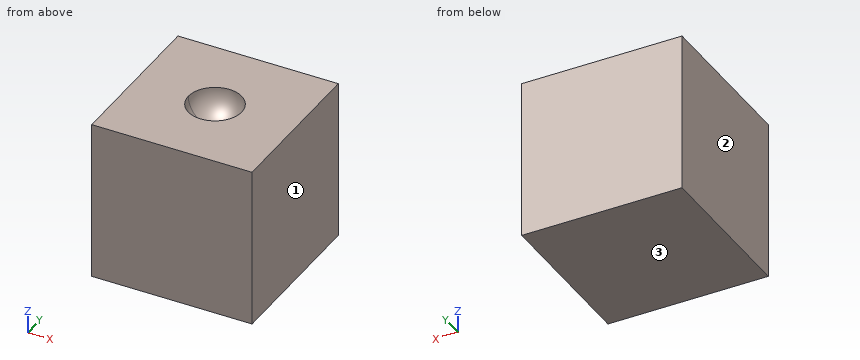
from build123d import *
from build123d.topology import SkipClean

# Parameters (mm, degrees)
SKETCH1_W           = 18
SKETCH1_H           = 18
BOSS_EXTRUDE1_DEPTH = 18


with BuildPart() as part:
    # Sketch1 → Boss-Extrude1 (new body)
    with BuildSketch(Plane.XY):
        Rectangle(SKETCH1_W, SKETCH1_H)
    extrude(amount=BOSS_EXTRUDE1_DEPTH)

    # Sketch2 → Cut-Revolve1 (revolve, cut)
    with SkipClean():  # the faces are left unmerged after this step: merging them gives an invalid solid
        with BuildSketch(Plane.XY.offset(18)):
            with BuildLine():
                ThreePointArc((3, 0), (2.121320344, 2.121320344), (0, 3))
                Line((0, 3), (0, -3))
                ThreePointArc((0, -3), (2.121320344, -2.121320344), (3, 0))
            make_face()
            with BuildLine():
                Line((0, -3), (0, 3))
                ThreePointArc((0, 3), (-3, 0), (0, -3))
            make_face()
        revolve(axis=Axis((0, 3, 18), (0, -1, 0)), mode=Mode.SUBTRACT)


solid = part.part
CAD build for the part. Positions are in the model's coordinates, mm. Face numbers are marked on the shaded views. Round coordinates to 2 decimals unless told otherwise and drop trailing zeros. Order: outer loops, then holes, each group sorted by start corner. A loop starts at its lowest first (then second) coordinate and runs counter-clockwise, first axis right, second up. Notation, with made-up numbers: (56, 1) -> (87, 1) arc R22 cw to (87, 11) -> close; hole circle Ø10 at (-2.5, 9.5). An arc over 180 degrees is marked (long way). Write each question's results on one line, items separated by ' | '.
1. Cut at A-A (z = 15.5). Give the cut face in (x, y).
Findings below:
outline: (-9, -9) -> (9, -9) -> (9, 9) -> (-9, 9) -> close; hole circle Ø3.32 at (0, 0)
2. Cut at B-B (x = 0.5). Give the cut face in (y, z).
Findings below:
outline: (-9, 0) -> (9, 0) -> (9, 18) -> (2.96, 18) arc R2.96 cw to (-2.96, 18) -> (-9, 18) -> close
3. Wall check: line 1 along X through (y, z) = (-2.5, 17.25); line 2 along Z through (x, y) = (-1.5, 1.5). Give the ranges that are in metal, low to high. Write a range as [from, to].
Findings below:
line 1: x = [-9, -1.48], [1.48, 9] | line 2: z = [0, 15.88]
4. Pull direction X, two halves, no side cores. Call the marked faces 1, 2 and 3: pulls with the +X half, pulls with the -X half, needs draft (parallel to the pull), parting line crosses it, or undercut.
Findings below:
face 1: pulls with the +X half | face 2: pulls with the -X half | face 3: needs draft
